Check sheet for the modelled part. Datum: model origin and axes. Units: mm. A direction names the side the tool comes from. Round coordinates to 2 decimals unless told otherwise and drop trailing zeros. Order: outer loops, then holes, each group sorted by start corner. A loop starts at its lowest first (then second) coordinate and runs counter-clockwise, first axis right, second up.
```python
from build123d import *

# Parameters (mm, degrees)
SKETCH_1_W          = 52.3
SKETCH_1_H          = 22.7
EXTRUDE_1_DEPTH     = 7.2
SKETCH_2_W          = 40.6
SKETCH_2_H          = 2.5
EXTRUDE_2_DEPTH     = 2
EXTRUDE_3_DEPTH     = 1
SKETCH_9_W          = 4
SKETCH_9_H          = 3
CUT_EXTRUDE_1_DEPTH = 3.6


with BuildPart() as part:
    # 草图1 → 凸台-拉伸1 (new body)
    with BuildSketch(Plane.XY):
        with Locations((-10.324857143, 4.54)):
            Rectangle(SKETCH_1_W, SKETCH_1_H)
    extrude(amount=EXTRUDE_1_DEPTH)

    # 草图2 → 凸台-拉伸2 (add)
    with BuildSketch(Plane(origin=(0, 0, 0), x_dir=(-1, 0, 0), z_dir=(0, 0, -1))):
        with Locations((10.674857143, -5.56)):
            Rectangle(SKETCH_2_W, SKETCH_2_H)
    extrude(amount=EXTRUDE_2_DEPTH)

    # 草图5 → 凸台-拉伸3 (add)
    with BuildSketch(Plane.ZY.offset(36.474857143)):
        with BuildLine():
            Line((4, 8.54), (4, 0.54))
            ThreePointArc((4, 0.54), (2.5, -0.96), (1, 0.54))
            Line((1, 0.54), (1, 8.54))
            ThreePointArc((1, 8.54), (2.5, 10.04), (4, 8.54))
        make_face()
    extrude(amount=EXTRUDE_3_DEPTH)

    # 草图9 → 切除-拉伸1 (cut)
    with BuildSketch(Plane.XY.offset(7.2)):
        with Locations((-25.474857143, -1.396404092)):
            Rectangle(SKETCH_9_W, SKETCH_9_H)
    extrude(amount=-CUT_EXTRUDE_1_DEPTH, mode=Mode.SUBTRACT)


solid = part.part
```
Item 1: Sectioned sample at C-C (x = -27). Record the cut outline in (y, z).
Answer:
outline: (-6.81, -2) - (-4.31, -2) - (-4.31, 0) - (15.89, 0) - (15.89, 7.2) - (0.1, 7.2) - (0.1, 3.6) - (-2.9, 3.6) - (-2.9, 7.2) - (-6.81, 7.2) - close
Item 2: Sectioned sample at A-A (z = 5). Record the cut outline in (x, y), and give its area (3 significant figures).
Answer:
outline: (-36.47, -6.81) - (15.83, -6.81) - (15.83, 15.89) - (-36.47, 15.89) - close; hole (-27.47, -2.9) - (-23.47, -2.9) - (-23.47, 0.1) - (-27.47, 0.1) - close
area: 1,180 mm2
Item 3: Sectioned sample at B-B (y = 2.75). Record the cut outline in (x, z), and give its area (3 significant figures).
Answer:
outline: (-37.47, 1) - (-36.47, 1) - (-36.47, 0) - (15.83, 0) - (15.83, 7.2) - (-36.47, 7.2) - (-36.47, 4) - (-37.47, 4) - close
area: 380 mm2
Item 4: Access from +Z, -Z, +X, -X, +Y, -Y to the whole of each face (thin tool, end or side, straight path). Record for faces 1 (the flat face through (-37, 5, 4)), 2 (the flat face through (-26, -1, 3.6)), 3 (the cylindrical face through (-36.97, -0.96, 2.53)).
Answer:
face 1: +Z, -X, +Y, -Y
face 2: +Z
face 3: -X, -Y
Item 5: Sectioned sample at D-D (z = -0.5). Record the cut outline in (x, y), and give its area (4 significant figures).
Answer:
outline: (-30.97, -6.81) - (9.63, -6.81) - (9.63, -4.31) - (-30.97, -4.31) - close
area: 101.5 mm2
Item 6: Go/stop test with flat-tipped pins: P1, Ø0.6, axis at y = -5.5, z = -0.5, coming from the -X side; P2, Ø0.5, axis at x = -37, y = 3, coming from the +Z side; P3, Ø0.5, axis at x = -37, y = 5, coming from the -Z side. Record where each tip stops, or that it passes through.
Answer:
P1: stops at x = -30.97
P2: stops at z = 4
P3: stops at z = 1
Item 7: Scan lines: line 1 along X through (y, z) = (-1.5, 5); line 2 along X through (y, z) = (10.75, 1.5); line 3 along Z through (x, y) = (0.5, -3). Record each from-to range of solid material in increasing order.
Answer:
line 1: x = -36.47 to -27.47, -23.47 to 15.83
line 2: x = -36.47 to 15.83
line 3: z = 0 to 7.2
Item 8: Release check for a two-part mould opening along Y. For faces 4 (the flat face through (-23.475, -1, 5)), 5 (the flat face through (-37, 4, 1)), 6 (the flat face through (-11, 15.89, 4)) record: released by +Y, released by -Y, zero draft, split by the parting line, or undercut.
Answer:
face 4: undercut
face 5: zero draft
face 6: released by +Y
